The drawing under review shows one solid part. Ordinate dimensions are in mm from its lowest x, y, z. A direction names the side the tool comes from. Give positions to 0.01 mm unless a question says otherwise; leave off trailing zeros. Loops run counter-clockwise (first coordinate to the right, second up) from the corner with the lowest first, then second, coordinate; pieces in that order, holes last. Notation, with made-up numbers: M 23,68 L 76,68 A31 cw 76,100 Z; hole C -28.75,42.25 d3. An arc over 180 degrees is marked long. One line per item, written item: value. Start each with the question number.
Q1. For pin 1 (2 mm diameter, centred on x = 62, z = 22, fed in from -Y); pin 2 (8 mm diameter, centred on x = 66, y = 74.5, fed in from -Z), all flat-tipped, find the tip position at first contact; note any pin that passes through.
Q2. We need section A-A on y = 8. Write out the cut boundary in (x, z).
Q3. To check wall thickness, follow line 1 along Y through (x, z) = (55.5, 17.75); line 2 along Y through (x, z) = (117.5, 5.5); line 3 along X through (y, z) = (49, 25). State the ranges of each line that lie inside material, in increasing order. Write a range as from..to.
Q4. We need section D-D on y = 87. Give the number of separate pieces and of enclosed holes in the cut face.
Q5. For the marked faces 5, 6 and 7, list the 3-axis set-ups (+Z, -Z, +X, -X, +Y, -Y) from which the entire face can be reached by the end or side of a thin tool; tool diameter is ignored.
Q6. Mouldability with a two-part tool opening along X and no side actions: class the marked faces 1, 2, 3 and 4 as released by +X, released by -X, zero draft, split by the parting line, or undercut.
Q7. We need section B-B on x = 87. Write out the cut boundary in (y, z), plus the area to 3 significant figures.
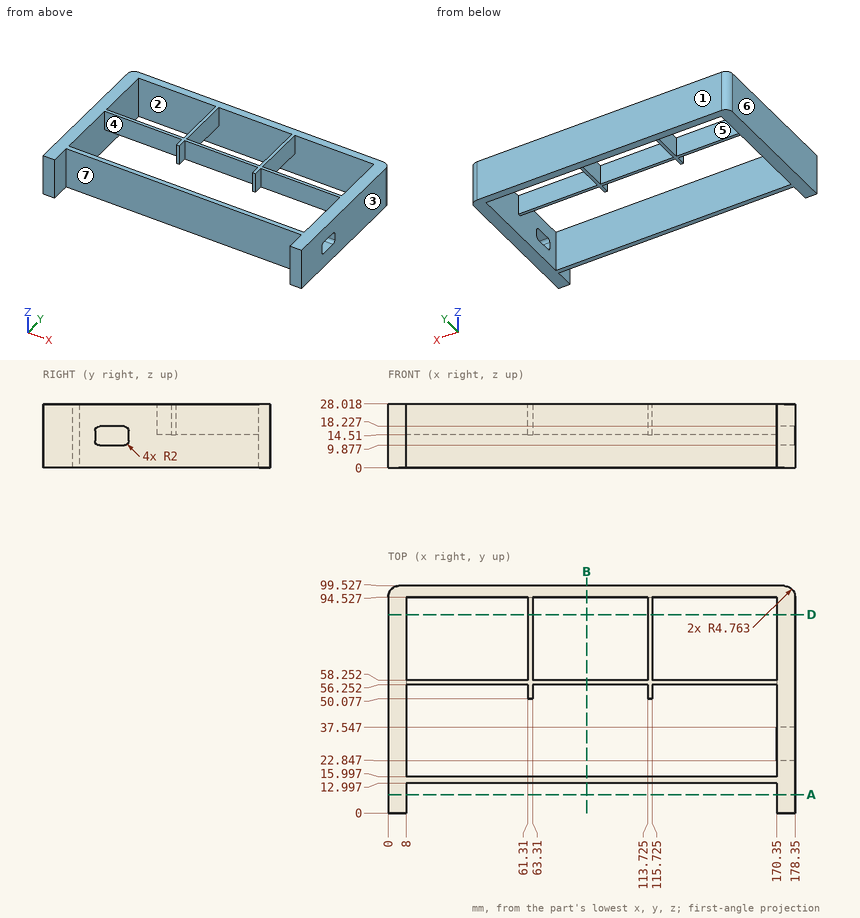
Solved:
1. pin 1: y = 13
1. pin 2: z = 14.51
2. outline: M 0,0 L 8,0 L 8,28.02 L 0,28.02 Z; M 170.35,0 L 178.35,0 L 178.35,28.02 L 170.35,28.02 Z
3. line 1: 13..16, 56.25..58.25, 94.53..99.53
3. line 2: 13..16, 94.53..99.53
3. line 3: 0..8, 170.35..178.35
4. separate pieces: 4
4. enclosed holes: 0
5. face 5: +Z, -Z
5. face 6: +Z, -Z, -X, +Y, -Y
5. face 7: +Z, -Z, -Y
6. face 1: zero draft
6. face 2: undercut
6. face 3: released by +X
6. face 4: undercut
7. outline: M 13,0 L 16,0 L 16,28.02 L 13,28.02 Z; M 56.25,14.51 L 58.25,14.51 L 58.25,28.02 L 56.25,28.02 Z; M 94.53,0 L 99.53,0 L 99.53,28.02 L 94.53,28.02 Z
7. area: 251 mm2
